Geometry check sheet. Reference: the model listing, model coordinates, mm. Face numbers are marked on the shaded views. A direction names the side the tool comes from. Give positions to 0.01 mm unless a question says otherwise; leave off trailing zeros. Write each loop counter-clockwise with the first axis right and the second up, starting at its lowest first coordinate (ties: lowest second). Pieces come first, ordered by that corner, then holes. Notation, with made-up numbers: (63, -1) -> (94, -1) arc R4 cw to (94, 4) -> close; hole circle Ø5 at (36.25, 50). An arc over 180 degrees is marked (long way). Write item = value, one per line. Start each with the question number.
1. Cross-section at B-B, the plane x = 1.5. Record the cut outline in (y, z) (3 decimals), plus the area to 3 significant figures.
2. Cross-section at C-C, the plane z = -4.5. Record the cut outline in (x, y) (3 decimals), plus the area to 3 significant figures.
3. Cross-section at A-A, the plane y = -14.3. Record the cut outline in (x, z), plus the area to 3 significant figures.
4. Mould release check, pull along Z, two halves, no side actions. Record for the marked faces 1, 2 and 3: pulls with the +Z half, pulls with the -Z half, needs draft (parallel to the pull), parting line crosses it, or undercut.
5. Cross-section at D-D, the plane y = -3. Record the cut outline in (x, z), plus the area to 3 significant figures.
6. Depth check by flat-ended pin: P1, Ø5.5, axis at x = 5.5, y = -13, coming from the +Z side; P2, Ø2, axis at x = 4, y = 12, coming from the -Z side; P3, Ø1, axis at x = 2.5, z = 7.5, coming from the -Y side (3 decimals); P4, Ø1.5, axis at x = 5.5, y = 13.5, coming from the -Z side. Enter the tip coordinate at first touch or a pass-through.
7. Thickness scan on line 1 along Y through (x, z) = (4.7, 6.1) (3 decimals); line 2 along Y through (x, z) = (4.7, 14.7) (3 decimals); line 3 along Y through (x, z) = (0.5, -11) (3 decimals). Record the ranges inside material, lowest first.
8. Set-up check for the marked faces 4, 5, 6 and 7: record each of +Z, -Z, +X, -X, +Y, -Y from which the full face is reachable in a straight line by a thin tool's end or side.
```python
from build123d import *

# Parameters (mm, degrees)
BOSS_EXTRUDE1_DEPTH = 9.4
FILLET1_R           = 0.5
FILLET2_R           = 0.5
SKETCH2_R           = 1
CUT_EXTRUDE1_DEPTH  = 27.98026362
SKETCH3_W           = 3.3
SKETCH3_H           = 1
BOSS_EXTRUDE2_DEPTH = 2.5
FILLET3_R           = 0.5
SKETCH4_R           = 2.435
SKETCH4_R_2         = 1
BOSS_EXTRUDE3_DEPTH = 3.2


with BuildPart() as part:
    # Sketch1 → Boss-Extrude1 (new body)
    with BuildSketch(Plane(origin=(0, 0, 0), x_dir=(0, 0, -1), z_dir=(1, 0, 0))):
        Polygon((-4.64, 11.565), (13.05, 11.565), (13.05, -11.565), (-4.64, -11.565), (-4.64, -16.055), (-6.49, -16.055), (-6.49, -11.565), (-13.05, -11.565), (-13.05, 11.565), (-6.49, 11.565), (-6.49, 16.055), (-4.64, 16.055), align=None)
    extrude(amount=BOSS_EXTRUDE1_DEPTH)

    # Fillet1
    fillet1_edges = [part.edges().sort_by_distance(p)[0] for p in [
        (0, -16.055, 5.565),
        (0, 16.055, 5.565),
        (9.4, 16.055, 5.565),
        (9.4, -16.055, 5.565),
    ]]
    fillet(fillet1_edges, radius=FILLET1_R)

    # Fillet2
    fillet2_edges = [part.edges().sort_by_distance(p)[0] for p in [
        (0, -11.565, -4.205),
        (0, -11.565, 9.77),
        (0, 0, 13.05),
        (0, 11.565, 9.77),
        (0, 11.565, -4.205),
        (0, 0, -13.05),
        (4.7, -11.565, -13.05),
        (4.7, -11.565, 13.05),
        (4.7, 11.565, 13.05),
        (4.7, 11.565, -13.05),
        (9.4, 11.565, 9.77),
        (9.4, 0, 13.05),
        (9.4, -11.565, 9.77),
        (9.4, -11.565, -4.205),
        (9.4, 0, -13.05),
        (9.4, 11.565, -4.205),
    ]]
    fillet(fillet2_edges, radius=FILLET2_R)

    # Sketch2 → Cut-Extrude1 (cut, through all)
    with BuildSketch(Plane.XY.offset(6.49)):
        with Locations((4.7, -14.3)):
            Circle(SKETCH2_R)
        with Locations((4.7, 14.3)):
            Circle(SKETCH2_R)
    extrude(amount=-CUT_EXTRUDE1_DEPTH, mode=Mode.SUBTRACT)

    # Sketch3 → Boss-Extrude2 (add)
    with BuildSketch(Plane(origin=(0, 11.565, 0), x_dir=(1, 0, 0), z_dir=(0, 1, 0))):
        with Locations((4.7, 9.470007)):
            Rectangle(SKETCH3_W, SKETCH3_H)
    extrude(amount=BOSS_EXTRUDE2_DEPTH)

    # Fillet3
    fillet3_edges = [part.edges().sort_by_distance(p)[0] for p in [
        (3.05, 14.065, -9.470007),
        (4.7, 14.065, -8.970007),
        (6.35, 14.065, -9.470007),
        (4.7, 14.065, -9.970007),
    ]]
    fillet(fillet3_edges, radius=FILLET3_R - 0.0001)  # a hair under: the kernel refuses the full size

    # Sketch4 → Boss-Extrude3 (add)
    with BuildSketch(Plane.XY.offset(13.05)):
        with Locations(Location((4.7, 6.88, 0), (0, 0, 180))):
            Circle(SKETCH4_R)
        with Locations((4.7, 6.88)):
            Circle(SKETCH4_R_2, mode=Mode.SUBTRACT)
    extrude(amount=BOSS_EXTRUDE3_DEPTH)


solid = part.part
```
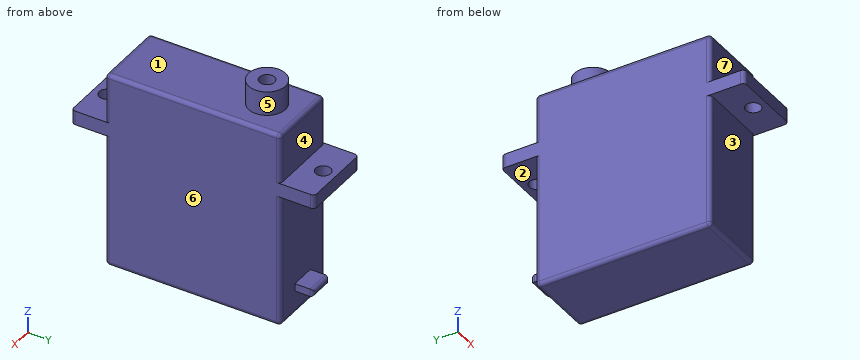
Answers:
q1.outline = (-16.055, 4.64) -> (-11.565, 4.64) -> (-11.565, -12.55) arc R0.5 ccw to (-11.065, -13.05) -> (11.065, -13.05) arc R0.5 ccw to (11.565, -12.55) -> (11.565, 4.64) -> (16.055, 4.64) -> (16.055, 6.49) -> (11.565, 6.49) -> (11.565, 12.55) arc R0.5 ccw to (11.065, 13.05) -> (-11.065, 13.05) arc R0.5 ccw to (-11.565, 12.55) -> (-11.565, 6.49) -> (-16.055, 6.49) -> close
q1.area = 620 mm^2
q2.outline = (0, -11.065) arc R0.5 ccw to (0.5, -11.565) -> (8.9, -11.565) arc R0.5 ccw to (9.4, -11.065) -> (9.4, 11.065) arc R0.5 ccw to (8.9, 11.565) -> (0.5, 11.565) arc R0.5 ccw to (0, 11.065) -> close
q2.area = 217 mm^2
q3.outline = (0, 4.64) -> (3.7, 4.64) -> (3.7, 6.49) -> (0, 6.49) -> close; (5.7, 4.64) -> (9.4, 4.64) -> (9.4, 6.49) -> (5.7, 6.49) -> close
q3.area = 13.7 mm^2
q4.face_1 = pulls with the +Z half
q4.face_2 = undercut
q4.face_3 = needs draft
q5.outline = (0, -12.55) arc R0.5 ccw to (0.5, -13.05) -> (8.9, -13.05) arc R0.5 ccw to (9.4, -12.55) -> (9.4, 12.55) arc R0.5 ccw to (8.9, 13.05) -> (0.5, 13.05) arc R0.5 ccw to (0, 12.55) -> close
q5.area = 245 mm^2
q6.P1 = 13.05
q6.P2 = -13.05
q6.P3 = -11.565
q6.P4 = -9.97
q7.line_1 = -16.055 to -15.3, -13.3 to 13.3, 15.3 to 16.055
q7.line_2 = 4.445 to 5.88, 7.88 to 9.315
q7.line_3 = -11.565 to 11.565
q8.face_4 = +Z, +X, -X, +Y
q8.face_5 = +Z
q8.face_6 = +Z, -Z, +X, +Y, -Y
q8.face_7 = +Z, +X, -X, -Y
